from build123d import *

# Parameters (mm, degrees)
SKETCH1_W               = 80
SKETCH1_H               = 40
BOSS_EXTRUDE1_DEPTH     = 20
SKETCH2_W               = 60
SKETCH2_H               = 7
CUT_EXTRUDE1_DEPTH      = 40
SKETCH3_W               = 14
SKETCH3_H               = 14
CUT_EXTRUDE2_DEPTH      = 80
CUT_EXTRUDE3_DEPTH      = 92.651513899
CUT_EXTRUDE3_DEPTH_BACK = 80
SKETCH4_R               = 4
SKETCH5_W               = 24
SKETCH5_H               = 24
CUT_EXTRUDE4_DEPTH      = 5
SKETCH6_R               = 10
CUT_EXTRUDE6_DEPTH      = 92.651513899


with BuildPart() as part:
    # Sketch1 → Boss-Extrude1 (new, symmetric)
    with BuildSketch(Plane.XY):
        with Locations((40, 20)):
            Rectangle(SKETCH1_W, SKETCH1_H)
    extrude(amount=BOSS_EXTRUDE1_DEPTH, both=True)

    # Sketch2 → Cut-Extrude1 (cut)
    with BuildSketch(Plane.XY.offset(20)):
        with Locations((40, 3.5)):
            Rectangle(SKETCH2_W, SKETCH2_H)
    extrude(amount=-CUT_EXTRUDE1_DEPTH, mode=Mode.SUBTRACT)

    # Sketch3 → Cut-Extrude2 (cut)
    with BuildSketch(Plane(origin=(80, 0, 0), x_dir=(0, 0, -1), z_dir=(1, 0, 0))):
        with Locations((0, 7)):
            Rectangle(SKETCH3_W, SKETCH3_H)
    extrude(amount=-CUT_EXTRUDE2_DEPTH, mode=Mode.SUBTRACT)

    # Sketch4 → Cut-Extrude3 (cut, two sides: drawn at the far end of the back side and taken through both)
    with BuildSketch(Plane(origin=(80, 0, 0), x_dir=(0, 0, -1), z_dir=(1, 0, 0)).offset(-CUT_EXTRUDE3_DEPTH_BACK)):
        with Locations(Location((0, 22, 0), (0, 0, 180))):
            Circle(SKETCH4_R)
    extrude(amount=CUT_EXTRUDE3_DEPTH + CUT_EXTRUDE3_DEPTH_BACK, mode=Mode.SUBTRACT)

    # Sketch5 → Cut-Extrude4 (cut)
    with BuildSketch(Plane(origin=(0, 40, 0), x_dir=(1, 0, 0), z_dir=(0, 1, 0))):
        with Locations((59, 0)):
            Rectangle(SKETCH5_W, SKETCH5_H)
        with Locations((21, 0)):
            Rectangle(SKETCH5_W, SKETCH5_H)
    extrude(amount=-CUT_EXTRUDE4_DEPTH, mode=Mode.SUBTRACT)

    # Sketch6 → Cut-Extrude6 (cut, through all)
    with BuildSketch(Plane(origin=(0, 40, 0), x_dir=(1, 0, 0), z_dir=(0, 1, 0))):
        with Locations(Location((59, 0, 0), (0, 0, 224.427004001))):
            Circle(SKETCH6_R)
        with Locations(Location((21, 0, 0), (0, 0, 224.427004001))):
            Circle(SKETCH6_R)
    extrude(amount=-CUT_EXTRUDE6_DEPTH, mode=Mode.SUBTRACT)


solid = part.part
Could you check a few things on this model? Use its own coordinates, in mm. A direction names the side the tool comes from. Give positions to 0.01 mm unless a question says otherwise; leave off trailing zeros. Order: outer loops, then holes, each group sorted by start corner. A loop starts at its lowest first (then second) coordinate and runs counter-clockwise, first axis right, second up. Notation, with made-up numbers: (22, 71.25) - (47, 71.25) arc R36 cw to (47, 106.25) - close; hole circle Ø4 at (-5.75, 63). An arc over 180 degrees is marked (long way). Return JSON: item names as keys, results as strings. Group by question number.
Q1. Please list where these lines run through material, in increasing order: line 1 along X through (y, z) = (34.5, -4); line 2 along X through (y, z) = (15, 0); line 3 along Z through (x, y) = (59, 22.25). Write a range as [from, to].
Q2. Suppose I cut it at A-A, the plane x = 59. Please give me the cut outline in (y, z), and give its area (3 significant figures).
Q3. Which directions (+Z, -Z, +X, -X, +Y, -Y) give clear straight access to the entire face, cutting with the end or side of a thin tool? Please do faces 1 (the face through (59, 38, 12)), 2 (the face through (5, 7, 7)), 3 (the face through (11.72, 24.31, 3.73)), 4 (the face through (40, 7, -13)).
Q4. Thinking about a two-plate mould opening in Y: for faces 5 (the face through (39, 40, 0)), 6 (the face through (39.862, 18.034, -0.521)), 7 (the face through (5, 7, -7)), 8 (the face through (40, 14, 0)), which applies, pulls with the +Y half, pulls with the -Y half, needs draft (parallel to the pull), parting line crosses it, or undercut?
Q5. Suppose I cut it at B-B, the plane y = 5. Please give me the cut outline in (x, z), and give its area (3 significant figures).
Q6. Suppose I cut it at C-C, the plane z = 0. State how many separate pieces and enclosed holes the cut face has, and give its area (3 significant figures).
Q7. Suppose I cut it at D-D, the plane x = 48. Please give me the cut outline in (y, z).
Q8. Will these pins go through, and if not, where does the flat tip stop? pin 1 Ø7 at (x, z) = (5, 1) entering from -Y; pin 2 Ø6.5 at (x, z) = (40, -11.5) entering from -Y.
Resolved:
{
 "1": {"line 1": "x = [0, 11.83], [30.17, 49.83], [68.17, 80]", "line 2": "x = [0, 11], [31, 49], [69, 80]", "line 3": "z = [-20, -10], [10, 20]"},
 "2": {"outline": "(7, -20) - (40, -20) - (40, -12) - (35, -12) - (35, -10) - (7, -10) - close; (7, 10) - (35, 10) - (35, 12) - (40, 12) - (40, 20) - (7, 20) - close", "area": "640 mm2"},
 "3": {"face 1": "+Y", "face 2": "+X, -X, -Y", "face 3": "+Y, -Y", "face 4": "+Z, -Z, -Y"},
 "4": {"face 5": "pulls with the +Y half", "face 6": "undercut", "face 7": "needs draft", "face 8": "pulls with the -Y half"},
 "5": {"outline": "(0, -20) - (10, -20) - (10, -7) - (0, -7) - close; (0, 7) - (10, 7) - (10, 20) - (0, 20) - close; (70, -20) - (80, -20) - (80, -7) - (70, -7) - close; (70, 7) - (80, 7) - (80, 20) - (70, 20) - close", "area": "520 mm2"},
 "6": {"separate pieces": "6", "enclosed holes": "0", "area": "680 mm2"},
 "7": {"outline": "(7, -20) - (40, -20) - (40, -12) - (35, -12) - (35, 12) - (40, 12) - (40, 20) - (7, 20) - (7, 7) - (14, 7) - (14, -7) - (7, -7) - close; hole circle Ø8 at (22, 0)"},
 "8": {"pin 1": "stops at y = 14", "pin 2": "stops at y = 7"}
}
